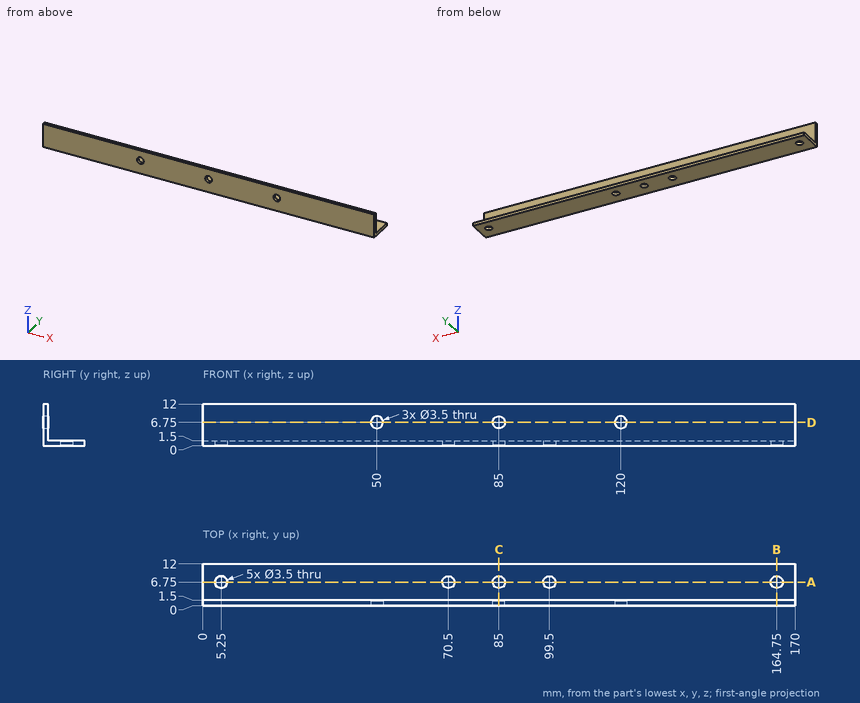
Drawing for the job (mm, zero at the part's lowest x, y, z). Round coordinates to 2 decimals unless told otherwise and drop trailing zeros. Write each loop counter-clockwise with the first axis right and the second up, starting at its lowest first coordinate (ties: lowest second). Pieces come first, ordered by that corner, then holes. Notation, with made-up numbers: M 38,4 L 65,4 A22 cw 65,38 Z; hole C 31,38.5 d6. An arc over 180 degrees is marked long. Answer in a Markdown table with one row per item.
1. Saw through at B-B (x = 164.75). List the corners of the cut face in (y, z).
Geometry check:
| item | result |
|---|---|
| outline | M 0,0 L 5,0 L 5,1.5 L 1.5,1.5 L 1.5,12 L 0,12 Z; M 8.5,0 L 12,0 L 12,1.5 L 8.5,1.5 Z |
2. Flat gauge pins, fed straight in: P1, Ø4.5, axis at x = 50, z = 6.75, coming from the +Y side; P2, Ø6, axis at x = 83, z = 9.5, coming from the -Y side; P3, Ø3, axis at x = 99.5, y = 6.75, coming from the -Z side; P4, Ø4, axis at x = 164.75, y = 6.75, coming from the +Z side. Where does each tip first touch, or does it go through?
Geometry check:
| item | result |
|---|---|
| P1 | y = 1.5 |
| P2 | y = 0 |
| P3 | through |
| P4 | z = 1.5 |
3. Saw through at C-C (x = 85). List the corners of the cut face in (y, z), and give its area (4 significant figures).
Geometry check:
| item | result |
|---|---|
| outline | M 0,0 L 5,0 L 5,1.5 L 1.5,1.5 L 1.5,5 L 0,5 Z; M 0,8.5 L 1.5,8.5 L 1.5,12 L 0,12 Z; M 8.5,0 L 12,0 L 12,1.5 L 8.5,1.5 Z |
| area | 23.25 mm2 |
4. Probe L1, parallel to X at y = 0.5, z = 7; L2, parallel to X at y = 6.75, z = 0.6; L3, parallel to Y at x = 85, z = 1.1. List the from-to ranges inside material, lowest first. Write a range as [from, to].
Geometry check:
| item | result |
|---|---|
| L1 | [0, 48.27], [51.73, 83.27], [86.73, 118.27], [121.73, 170] |
| L2 | [0, 3.5], [7, 68.75], [72.25, 83.25], [86.75, 97.75], [101.25, 163], [166.5, 170] |
| L3 | [0, 5], [8.5, 12] |
5. Saw through at A-A (y = 6.75). List the corners of the cut face in (x, z), and give its area (3 significant figures).
Geometry check:
| item | result |
|---|---|
| outline | M 0,0 L 3.5,0 L 3.5,1.5 L 0,1.5 Z; M 7,0 L 68.75,0 L 68.75,1.5 L 7,1.5 Z; M 72.25,0 L 83.25,0 L 83.25,1.5 L 72.25,1.5 Z; M 86.75,0 L 97.75,0 L 97.75,1.5 L 86.75,1.5 Z; M 101.25,0 L 163,0 L 163,1.5 L 101.25,1.5 Z; M 166.5,0 L 170,0 L 170,1.5 L 166.5,1.5 Z |
| area | 229 mm2 |
6. Saw through at D-D (z = 6.75). List the corners of the cut face in (x, y).
Geometry check:
| item | result |
|---|---|
| outline | M 0,0 L 48.25,0 L 48.25,1.5 L 0,1.5 Z; M 51.75,0 L 83.25,0 L 83.25,1.5 L 51.75,1.5 Z; M 86.75,0 L 118.25,0 L 118.25,1.5 L 86.75,1.5 Z; M 121.75,0 L 170,0 L 170,1.5 L 121.75,1.5 Z |
